Can you work these out from the drawing? Everything is in mm from the part's minimum corner. A direction names the side the tool comes from. Coordinates: 2 decimals unless noted, no trailing zeros. Write each loop counter-clockwise with the first axis right and the second up, starting at its lowest first coordinate (ties: lowest second). Pieces come first, ordered by that corner, then holes.
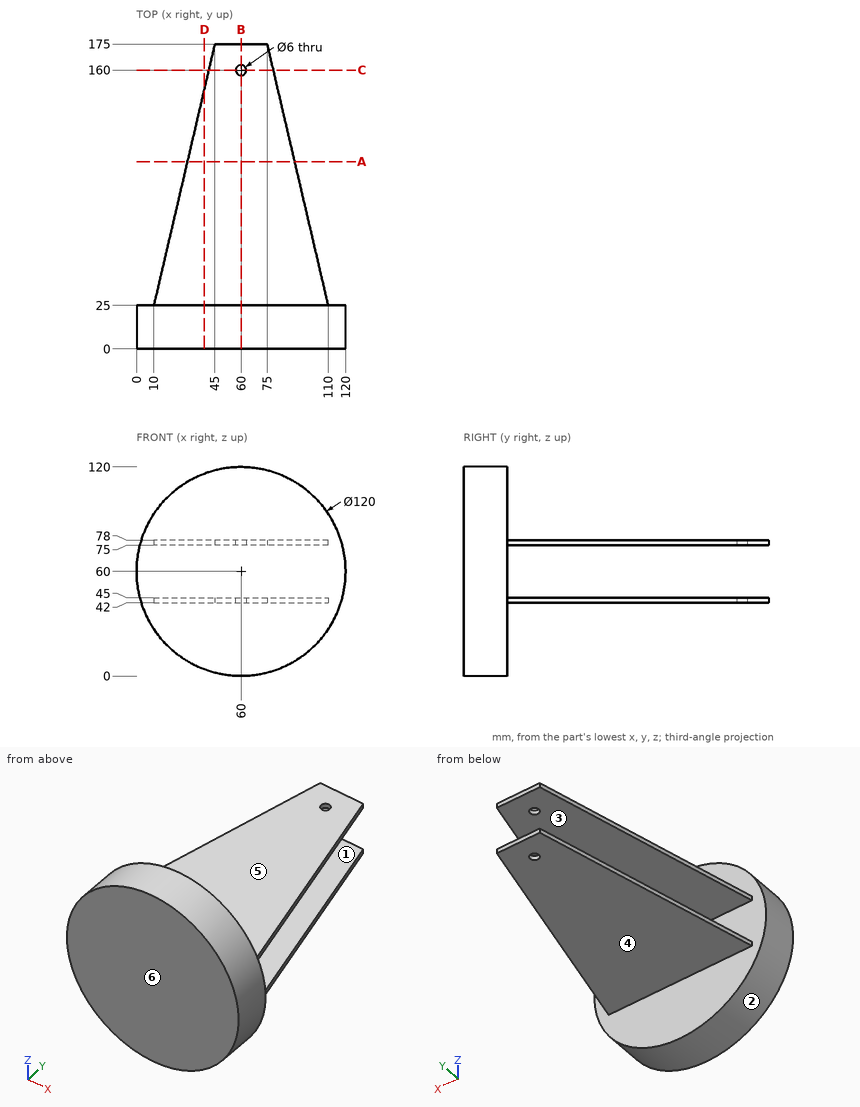
1. I want a section at A-A (y = 107.5). List the corners of the cut face in (x, z) for me.
2. If I drill on line 1 (Y direction, x = 60, z = 77.2); line 2 (Z direction, x = 40.5, y = 150); line 3 (Y direction, x = 21, z = 96), over which ranges is the centre line in solid material (lowest first)?
3. I want a section at D-D (x = 39). List the corners of the cut face in (y, z) for me, then the cut area to 3 significant figures.
4. Thinking about a two-plate mould opening in Z: for the marked faces 3, 4, 5 and 6, which applies, pulls with the +Z half, pulls with the -Z half, needs draft (parallel to the pull), parting line crosses it, or undercut?
5. On a 3-axis mill with a long thin cutter (end or side, diameter ignored), from which of +Z, -Z, +X, -X, +Y, -Y can I reach the whole of each face in a straight line? I mean the marked faces 1 and 2. Say none if no direction works.
6. For pin 1 Ø2 at (x, z) = (43, 54) entering from -Y; pin 2 Ø3 at (x, y) = (47, 19.5) entering from -Z; pin 3 Ø12 at (x, y) = (47, 121) entering from +Z; pin 4 Ø3.5 at (x, y) = (60, 160) entering from -Z, each with a flat end and sliding along its axis, tell me the tip position at first contact or that it passes through.
7. I want a section at B-B (x = 60). List the corners of the cut face in (y, z) for me, then the cut area to 3 significant figures.
8. I want a section at C-C (y = 160). List the corners of the cut face in (x, z) for me.
Response values:
1. outline: (29.25, 42) - (90.75, 42) - (90.75, 45) - (29.25, 45) - close; (29.25, 75) - (90.75, 75) - (90.75, 78) - (29.25, 78) - close
2. line 1: y = 0 to 157, 163 to 175
2. line 2: z = 42 to 45, 75 to 78
2. line 3: y = 0 to 25
3. outline: (0, 3.8) - (25, 3.8) - (25, 42) - (149.29, 42) - (149.29, 45) - (25, 45) - (25, 75) - (149.29, 75) - (149.29, 78) - (25, 78) - (25, 116.2) - (0, 116.2) - close
3. area: 3,560 mm2
4. face 3: undercut
4. face 4: pulls with the -Z half
4. face 5: pulls with the +Z half
4. face 6: needs draft
5. face 1: +X, -X, +Y
5. face 2: +Y, -Y
6. pin 1: stops at y = 0
6. pin 2: stops at z = 1.11
6. pin 3: stops at z = 78
6. pin 4: passes through
7. outline: (0, 0) - (25, 0) - (25, 42) - (157, 42) - (157, 45) - (25, 45) - (25, 75) - (157, 75) - (157, 78) - (25, 78) - (25, 120) - (0, 120) - close; (163, 42) - (175, 42) - (175, 45) - (163, 45) - close; (163, 75) - (175, 75) - (175, 78) - (163, 78) - close
7. area: 3,860 mm2
8. outline: (41.5, 42) - (57, 42) - (57, 45) - (41.5, 45) - close; (41.5, 75) - (57, 75) - (57, 78) - (41.5, 78) - close; (63, 42) - (78.5, 42) - (78.5, 45) - (63, 45) - close; (63, 75) - (78.5, 75) - (78.5, 78) - (63, 78) - close
